Geometry check sheet. Reference: drawing and pictorial views, mm from the part's lowest x, y, z. A direction names the side the tool comes from. Give positions to 0.01 mm unless a question says otherwise; leave off trailing zeros. Write each loop counter-clockwise with the first axis right and the second up, starting at its lowest first coordinate (ties: lowest second). Pieces come first, ordered by that corner, then holes. Notation, with made-up numbers: (-14, 40) -> (42, 40) arc R25 ccw to (42, 70) -> close; hole circle Ø3 at (62, -28). An arc over 180 degrees is marked (long way). Answer as CSV lines item,"result".
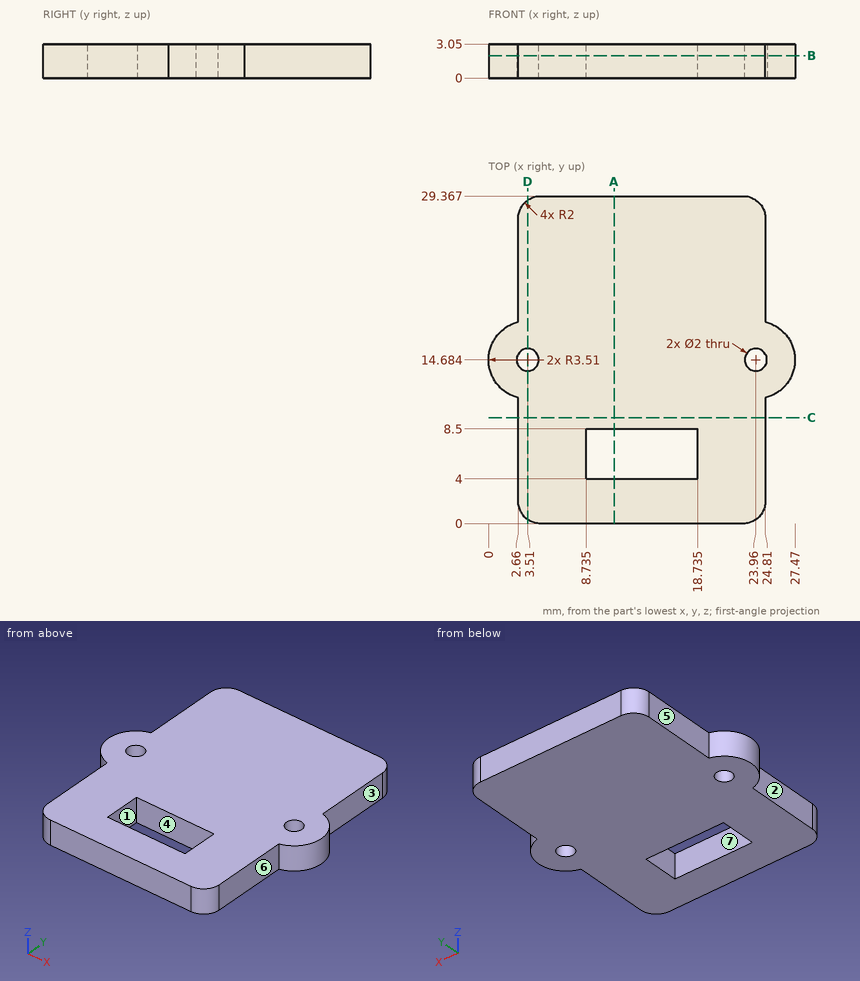
1) Scan lines: line 1 along X through (y, z) = (4.25, 1.2) (1 decimal); line 2 along Y through (x, z) = (17.25, 0.9); line 3 along X through (y, z) = (15.5, 1.3) (1 decimal). Record each from-to range of solid material in increasing order.
Reported:
line 1,"2.7 to 8.7, 18.7 to 24.8"
line 2,"0 to 4, 8.5 to 29.37"
line 3,"0.1 to 2.9, 4.1 to 23.4, 24.5 to 27.4"
2) Section check D-D (x = 3.51). Record the boundary of the cut face in (y, z).
Reported:
outline,"(0.36, 0) -> (13.68, 0) -> (13.68, 3.05) -> (0.36, 3.05) -> close; (15.68, 0) -> (29, 0) -> (29, 3.05) -> (15.68, 3.05) -> close"
3) Section check A-A (x = 11.25). Record the boundary of the cut face in (y, z).
Reported:
outline,"(0, 0) -> (4, 0) -> (4, 3.05) -> (0, 3.05) -> close; (8.5, 0) -> (29.37, 0) -> (29.37, 3.05) -> (8.5, 3.05) -> close"
4) Section check B-B (z = 2). Record the boundary of the cut face in (x, y) (1 decimal).
Reported:
outline,"(2.7, 2) arc R2 ccw to (4.7, 0) -> (22.8, 0) arc R2 ccw to (24.8, 2) -> (24.8, 11.3) arc R3.5 ccw to (24.8, 18.1) -> (24.8, 27.4) arc R2 ccw to (22.8, 29.4) -> (4.7, 29.4) arc R2 ccw to (2.7, 27.4) -> (2.7, 18.1) arc R3.5 ccw to (2.7, 11.3) -> close; hole circle Ø2 at (3.5, 14.7); hole (8.7, 4) -> (18.7, 4) -> (18.7, 8.5) -> (8.7, 8.5) -> close; hole circle Ø2 at (24, 14.7)"
5) Tool access check on the marked faces 5, 6 and 7. Record the directions out of +Z, -Z, +X, -X, +Y, -Y that give a thin tool (end or side, any length) a straight path to the whole face; none if there is none.
Reported:
face 5,"+Z, -Z, -X, +Y"
face 6,"+Z, -Z, +X, -Y"
face 7,"+Z, -Z"
6) Section check C-C (y = 9.5). Record the boundary of the cut face in (x, z).
Reported:
outline,"(2.66, 0) -> (24.81, 0) -> (24.81, 3.05) -> (2.66, 3.05) -> close"
7) Draft check along X on the marked faces 1, 2, 3 and 4. Enter one of: +X half, -X half, draft (parallel to the pull), parting line (faces both ways), or undercut.
Reported:
face 1,"undercut"
face 2,"-X half"
face 3,"+X half"
face 4,"undercut"
8) Depth check by flat-ended pin: pin 1 (1.2 mm diameter, centred on x = 3.51, y = 14.68, fed in from +Z); pin 2 (0.9 mm diameter, centred on y = 5.5, z = 1, fed in from +X); pin 3 (1.5 mm diameter, centred on y = 8.5, z = 1, fed in from -X). Enter the tip coordinate at first touch or a pass-through.
Reported:
pin 1,"through"
pin 2,"x = 24.81"
pin 3,"x = 2.66"
